Part print with two shaded views. Sizes in mm from the minimum x, y, z corner. A direction names the side the tool comes from. Coordinates: 2 decimals unless noted, no trailing zeros. Loops run counter-clockwise (first coordinate to the right, second up) from the corner with the lowest first, then second, coordinate; pieces in that order, holes last. Notation, with made-up numbers: (35.25, 54.25) -> (55.25, 54.25) arc R6 ccw to (55.25, 60.25) -> close; hole circle Ø7 at (63.5, 61.25). An arc over 180 degrees is marked (long way). Return JSON: item names as keys, results as strings. Group by question number.
(1) Saw through at A-A on x = 3. Write the cut outline in (y, z).
(2) Saw through at C-C on y = 6.5. Write the cut outline in (x, z).
(3) Tool access for the marked faces 1 and 2: list every direction of +Z, -Z, +X, -X, +Y, -Y with a clear straight run to the whole face (end or side of a thin tool).
(4) Saw through at B-B on z = 3.25. Write the cut outline in (x, y).
(5) Saw through at D-D on x = 4. Write the cut outline in (y, z), then the cut area to 3 significant figures.
(6) Probe L1, parallel to Z at x = 3.1, y = 2.75; L2, parallel to Y at x = 1.6, z = 1.25; L3, parallel to X at y = 11, z = 5. List the from-to ranges inside material, lowest first.
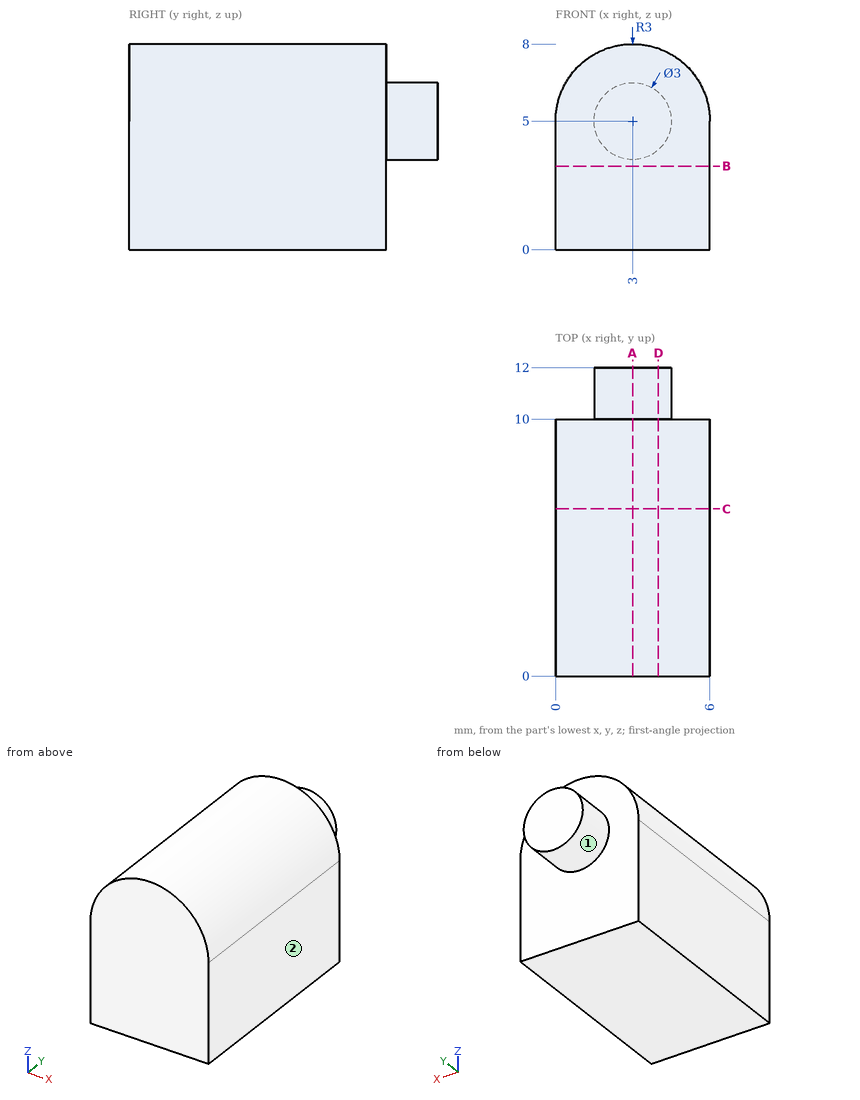
Geometry results:
{
 "1": {"outline": "(0, 0) -> (10, 0) -> (10, 3.5) -> (12, 3.5) -> (12, 6.5) -> (10, 6.5) -> (10, 8) -> (0, 8) -> close"},
 "2": {"outline": "(0, 0) -> (6, 0) -> (6, 5) arc R3 ccw to (0, 5) -> close"},
 "3": {"face 1": "+Y", "face 2": "+Z, -Z, +X, +Y, -Y"},
 "4": {"outline": "(0, 0) -> (6, 0) -> (6, 10) -> (0, 10) -> close"},
 "5": {"outline": "(0, 0) -> (10, 0) -> (10, 3.88) -> (12, 3.88) -> (12, 6.12) -> (10, 6.12) -> (10, 7.83) -> (0, 7.83) -> close", "area": "82.8 mm²"},
 "6": {"L1": "0 to 8", "L2": "0 to 10", "L3": "1.5 to 4.5"}
}
